```python
from build123d import *

# Parameters (mm, degrees)
F0_W     = 7
F0_H     = 18
F0_R     = 2
F0_W_2   = 10
F1_DEPTH = 8
F3_D     = 3.4
F4_W     = 9
F4_H     = 3.2
F5_DEPTH = 25
F6_DEPTH = 2
F7_DEPTH = 2
F8_R     = 2
F9_DEPTH = 4
F10_R    = 3.99999


# Not quite as in the source:
# - a fillet or chamfer is up to 0.001 mm smaller than in the source, because OpenCascade refuses the exact size


with BuildPart() as f1:
    # F0 (on Top) → F1 (new body)
    with BuildSketch(Plane.XY):
        with Locations((-1.6666666667, 0)):
            Rectangle(F0_W, F0_H)
        with Locations((-2.1666666667, -4)):
            Circle(F0_R, mode=Mode.SUBTRACT)
        with Locations((-2.1666666667, 4)):
            Circle(F0_R, mode=Mode.SUBTRACT)
        with Locations((6.8333333333, 0)):
            Rectangle(F0_W_2, F0_H)
    extrude(amount=F1_DEPTH)

    # F3 (through all)
    with Locations(Plane.XZ.offset(9)):
        with Locations((7.8333333333, 4)):
            Hole(F3_D / 2)

    # F4 (on face) → F5 (cut)
    with BuildSketch(Plane.XY.offset(8)):
        with Locations((7.3333333333, 6.2)):
            Rectangle(F4_W, F4_H)
        with Locations((7.3333333333, 0)):
            Rectangle(F4_W, F4_H)
        with Locations((7.3333333333, -6.2)):
            Rectangle(F4_W, F4_H)
    extrude(amount=-F5_DEPTH, mode=Mode.SUBTRACT)

    # F6 (add): a face of the model
    f6_faces = [f1.faces().sort_by_distance(p)[0] for p in [
        (3.0114285443, -9, 4),
    ]]
    extrude(f6_faces, amount=F6_DEPTH)

    # F7 (add): a face of the model
    f7_faces = [f1.faces().sort_by_distance(p)[0] for p in [
        (3.0114285443, 9, 4),
    ]]
    extrude(f7_faces, amount=F7_DEPTH)

    # F8 (on face) → F9 (cut)
    with BuildSketch(Plane(origin=(0, 0, 0), x_dir=(1, 0, 0), z_dir=(0, 0, -1))):
        Polygon((2.8333333333, 7.8), (2.8333333333, 11), (-5.1666666667, 11), (-5.1666666667, -11), (2.8333333333, -11), (2.8333333333, -7.8), (2.8333333333, -4.6), (2.8333333333, -1.6), (2.8333333333, 1.6), (2.8333333333, 4.6), align=None)
        with Locations((-2.1666666667, -4)):
            Circle(F8_R, mode=Mode.SUBTRACT)
        with Locations((-2.1666666667, 4)):
            Circle(F8_R, mode=Mode.SUBTRACT)
    extrude(amount=-F9_DEPTH, mode=Mode.SUBTRACT)

    # F10 (radius 4 in the source; OpenCascade refuses exactly that, so slightly less here)
    f10_edges = [f1.edges().sort_by_distance(p)[0] for p in [
        (-5.166667, -11, 6),
        (-5.166667, 11, 6),
        (2.833333, -9.4, 0),
        (2.833333, -3.1, 0),
        (2.833333, 3.1, 0),
        (2.833333, 9.4, 0),
        (11.833333, -9.4, 0),
        (11.833333, -3.1, 0),
        (11.833333, 3.1, 0),
        (11.833333, 9.4, 0),
    ]]
    fillet(f10_edges, radius=F10_R)


solid = f1.part
```
Check sheet for the modelled part. Datum: model origin and axes. Units: mm. A direction names the side the tool comes from. Round coordinates to 2 decimals unless told otherwise and drop trailing zeros. Order: outer loops, then holes, each group sorted by start corner. A loop starts at its lowest first (then second) coordinate and runs counter-clockwise, first axis right, second up. Notation, with made-up numbers: (-25.5, 10) -> (12.5, 10) arc R28 ccw to (12.5, 45) -> close; hole circle Ø2 at (4.25, -39). An arc over 180 degrees is marked (long way). One line per item, written item: value. Start each with the question number.
Q1. Mould release check, pull along X, two halves, no side actions. Record for faces 3 (the face through (7, 3, 0)), 4 (the face through (-0.32, -4.77, 5.97)), 5 (the face through (3.974, -9.422, 1.203)): pulls with the +X half, pulls with the -X half, needs draft (parallel to the pull), parting line crosses it, or undercut.
Q2. Thickness scan on line 1 (Y direction, x = 3, z = 7.75); line 2 (Z direction, x = -1.75, y = -9.25); line 3 (X direction, y = -4, z = 5). Record the ranges inside material, lowest first.
Q3. Set-up check for faces 1 (the face through (-4.026, -9.797, 6.028)), 2 (the face through (2.833, -6, 6)): record each of +Z, -Z, +X, -X, +Y, -Y from which the full face is reachable in a straight line by a thin tool's end or side.
Q4. Cross-section at A-A (y = 4). Give the number of separate pieces and of enclosed holes in the cut face, and give its area (3 significant figures).
Q5. Gauge pin test, flat ends, axial feed: pin 1 Ø2.5 at (y, z) = (6.5, 6.5) entering from +X; pin 2 Ø2.5 at (x, y) = (0.5, 4) entering from -Z; pin 3 Ø3 at (y, z) = (-2.5, 1.5) entering from +X. Record the tip position at first contact, or that the pin passes through.
Q6. Cross-section at C-C (x = 5). Record the boundary of the cut face in (y, z), and give its area (3 significant figures).
Completed:
1. face 3: needs draft
1. face 4: undercut
1. face 5: pulls with the -X half
2. line 1: y = -11 to -7.8, -4.6 to -1.6, 1.6 to 4.6, 7.8 to 11
2. line 2: z = 4 to 8
2. line 3: x = -5.17 to -4.17, -0.17 to 6.46, 9.21 to 11.83
3. face 1: +Z, -Z, -X, -Y
3. face 2: +Z, -Z, +X
4. separate pieces: 2
4. enclosed holes: 1
4. area: 72.1 mm²
5. pin 1: stops at x = 2.83
5. pin 2: stops at z = 4
5. pin 3: stops at x = 11.71
6. outline: (-11, 0.44) -> (-7.8, 0.44) -> (-7.8, 8) -> (-11, 8) -> close; (-4.6, 0.44) -> (-1.6, 0.44) -> (-1.6, 8) -> (-4.6, 8) -> close; (1.6, 0.44) -> (4.6, 0.44) -> (4.6, 8) -> (1.6, 8) -> close; (7.8, 0.44) -> (11, 0.44) -> (11, 8) -> (7.8, 8) -> close
6. area: 93.7 mm²
